Geometry: final body of the model. Coordinates: model frame, mm. Give positions to 0.01 mm unless a question says otherwise; leave off trailing zeros. Write each loop counter-clockwise with the first axis right and the second up, starting at its lowest first coordinate (ties: lowest second). Pieces come first, ordered by that corner, then holes. Notation, with made-up numbers: (20, -1) -> (69, -1) arc R18 cw to (69, 22) -> close; hole circle Ø2 at (33, 54). An arc over 180 degrees is marked (long way). Answer in a Markdown table with one row per item. Add a question column.
Item 1: Material intervals for probe 1 along Z at (x, y) = (24.8, -6.05); probe 2 along Y at (x, z) = (0, 204.25); probe 3 along Z at (x, y) = (1.5, -5.25), sorted ascending. Write a range as from..to.
Item 2: First-contact query: P1, Ø2, axis at x = 10.5, y = -5.5, coming from the +Z side; P2, Ø1.8, axis at x = 0, y = 0, coming from the -Z side; P3, Ø2.5, axis at x = 24.8, y = 0, coming from the +Z side; P4, Ø1.5, axis at y = -5, z = 119, coming from the +X side. Flat tips, straight axial feed; report the tip coordinate or a pass-through.
Item 3: Section query A-A on z = 43. Output: boundary loops of the cut face in (x, y).
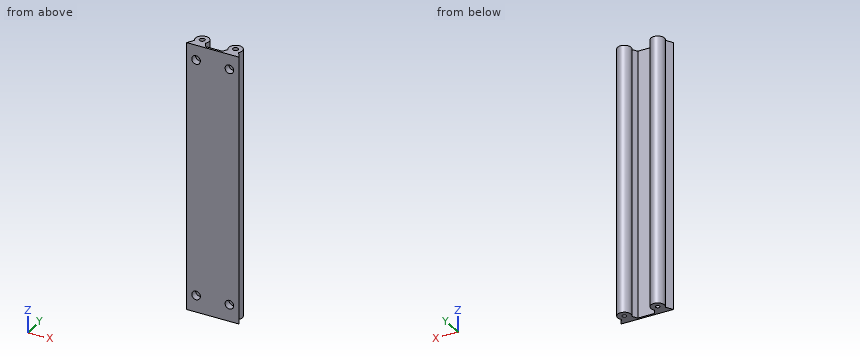
```python
from build123d import *

# Parameters (mm, degrees)
SKETCH1_R           = 5
BOSS_EXTRUDE1_DEPTH = 220
BOSS_EXTRUDE4_DEPTH = 220
SKETCH5_R           = 1.37
CUT_EXTRUDE1_DEPTH  = 7
SKETCH6_R           = 1.37
CUT_EXTRUDE2_DEPTH  = 7
CUT_EXTRUDE4_DEPTH  = 10.8
CUT_EXTRUDE5_DEPTH  = 10.8
SKETCH11_R          = 2
CUT_EXTRUDE6_DEPTH  = 7
SKETCH12_R          = 1.5
CUT_EXTRUDE7_DEPTH  = 7
SKETCH4_R           = 3.2
CUT_EXTRUDE9_DEPTH  = 5


with BuildPart() as part:
    # Sketch1 → Boss-Extrude1 (new body)
    with BuildSketch(Plane.XY):
        Circle(SKETCH1_R)
        with BuildLine():
            Line((-4, -3), (-7, -8.196152423))
            Line((-7, -8.196152423), (7, -8.196152423))
            Line((7, -8.196152423), (4, -3))
            ThreePointArc((4, -3), (0, 5), (-4, -3))
        make_face()
        with BuildLine():
            Line((28.8, -3), (31.8, -8.196152423))
            Line((31.8, -8.196152423), (17.8, -8.196152423))
            Line((17.8, -8.196152423), (20.8, -3))
            ThreePointArc((20.8, -3), (24.8, 5), (28.8, -3))
        make_face()
    extrude(amount=BOSS_EXTRUDE1_DEPTH)

    # Sketch3 → Boss-Extrude4 (add)
    with BuildSketch(Plane.XY.offset(220)):
        Polygon((7, -8.196152423), (17.8, -8.196152423), (18.65, -8.196152423), (18.65, -6.723909236), (6.15, -6.723909236), (6.15, -8.196152423), align=None)
    extrude(amount=-BOSS_EXTRUDE4_DEPTH)

    # Sketch5 → Cut-Extrude1 (cut)
    with BuildSketch(Plane(origin=(0, 0, 0), x_dir=(-1, 0, 0), z_dir=(0, 0, -1))):
        Circle(SKETCH5_R)
        with Locations((-24.8, 0)):
            Circle(SKETCH5_R)
    extrude(amount=-CUT_EXTRUDE1_DEPTH, mode=Mode.SUBTRACT)

    # Sketch6 → Cut-Extrude2 (cut)
    with BuildSketch(Plane.XY.offset(220)):
        Circle(SKETCH6_R)
        with Locations((24.8, 0)):
            Circle(SKETCH6_R)
    extrude(amount=-CUT_EXTRUDE2_DEPTH, mode=Mode.SUBTRACT)

    # Sketch9 → Cut-Extrude4 (cut)
    with BuildSketch(Plane(origin=(0, 0, 0), x_dir=(-1, 0, 0), z_dir=(0, 0, -1))):
        with BuildLine():
            Line((-28.8, -3), (-31.8, -8.196152423))
            Line((-31.8, -8.196152423), (7, -8.196152423))
            Line((7, -8.196152423), (4, -3))
            ThreePointArc((4, -3), (0, 5), (-4, -3))
            Line((-4, -3), (-6.15, -6.723909236))
            Line((-6.15, -6.723909236), (-18.65, -6.723909236))
            Line((-18.65, -6.723909236), (-20.8, -3))
            ThreePointArc((-20.8, -3), (-24.8, 5), (-28.8, -3))
        make_face()
    extrude(amount=-CUT_EXTRUDE4_DEPTH, mode=Mode.SUBTRACT)

    # Sketch10 → Cut-Extrude5 (cut)
    with BuildSketch(Plane.XY.offset(220)):
        with BuildLine():
            Line((20.8, -3), (18.65, -6.723909236))
            Line((18.65, -6.723909236), (6.15, -6.723909236))
            Line((6.15, -6.723909236), (4, -3))
            ThreePointArc((4, -3), (0, 5), (-4, -3))
            Line((-4, -3), (-7, -8.196152423))
            Line((-7, -8.196152423), (31.8, -8.196152423))
            Line((31.8, -8.196152423), (28.8, -3))
            ThreePointArc((28.8, -3), (24.8, 5), (20.8, -3))
        make_face()
    extrude(amount=-CUT_EXTRUDE5_DEPTH, mode=Mode.SUBTRACT)

    # Sketch11 → Cut-Extrude6 (cut)
    with BuildSketch(Plane.XY.offset(209.2)):
        Circle(SKETCH11_R)
        with Locations((24.8, 0)):
            Circle(SKETCH11_R)
    extrude(amount=-CUT_EXTRUDE6_DEPTH, mode=Mode.SUBTRACT)

    # Sketch12 → Cut-Extrude7 (cut)
    with BuildSketch(Plane(origin=(0, 0, 10.8), x_dir=(-1, 0, 0), z_dir=(0, 0, -1))):
        Circle(SKETCH12_R)
        with Locations((-24.8, 0)):
            Circle(SKETCH12_R)
    extrude(amount=-CUT_EXTRUDE7_DEPTH, mode=Mode.SUBTRACT)

    # Sketch4 → Cut-Extrude9 (cut)
    with BuildSketch(Plane.XZ.offset(8.196152423)):
        with Locations((0, 23.2)):
            Circle(SKETCH4_R)
        with Locations((24.8, 23.2)):
            Circle(SKETCH4_R)
        with Locations((0, 198.2)):
            Circle(SKETCH4_R)
        with Locations((24.8, 198.2)):
            Circle(SKETCH4_R)
    extrude(amount=-CUT_EXTRUDE9_DEPTH, mode=Mode.SUBTRACT)


solid = part.part
```
Findings below:
| question | item | result |
|---|---|---|
| 1 | probe 1 | z = 10.8..20, 26.4..195, 201.4..209.2 |
| 1 | probe 2 | y = -8.2..-2, 2..5 |
| 1 | probe 3 | z = 10.8..20.37, 26.03..195.37, 201.03..209.2 |
| 2 | P1 | passes through |
| 2 | P2 | stops at z = 17.8 |
| 2 | P3 | stops at z = 202.2 |
| 2 | P4 | stops at x = 30.39 |
| 3 | outline | (-7, -8.2) -> (31.8, -8.2) -> (28.8, -3) arc R5 ccw (long way) to (20.8, -3) -> (18.65, -6.72) -> (6.15, -6.72) -> (4, -3) arc R5 ccw (long way) to (-4, -3) -> close |
